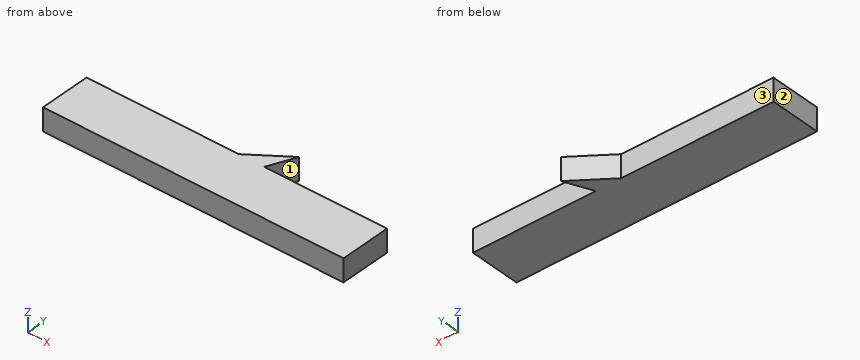
from build123d import *

# Parameters (mm, degrees)
F1_DEPTH = 25


with BuildPart() as f1:
    # F0 (on Top) → F1 (new body)
    with BuildSketch(Plane.XY):
        Polygon((-143.368647, 7.681685), (-52.16566, 7.681685), (25.298358, 63.81616), (-143.368647, 63.81616), align=None)
        Polygon((25.298358, 63.81616), (-52.16566, 7.681685), (189.367071, 7.681685), (189.367071, 63.81616), (53.402534, 63.81616), align=None)
        Polygon((66.434935, 93.625873), (25.298358, 63.81616), (53.402534, 63.81616), align=None)
    extrude(amount=F1_DEPTH)


solid = f1.part
Geometry check sheet. Reference: the model listing, model coordinates, mm. Face numbers are marked on the shaded views. Round coordinates to 2 decimals unless told otherwise and drop trailing zeros. Write each loop counter-clockwise with the first axis right and the second up, starting at its lowest first coordinate (ties: lowest second). Pieces come first, ordered by that corner, then holes. Notation, with made-up numbers: (44.25, 34.5) - (63.25, 34.5) arc R13 cw to (63.25, 55.5) - close; hole circle Ø8 at (56, 83.25). An arc over 180 degrees is marked (long way). One line per item, written item: value.
1. Cross-section at D-D on y = 68. Record the boundary of the cut face in (x, z), and give its area (3 significant figures).
The answers:
outline: (31.07, 0) - (55.23, 0) - (55.23, 25) - (31.07, 25) - close
area: 604 mm^2
2. Scan lines: L1, parallel to Y at x = -62.5, z = 11.25; L2, parallel to X at y = 77, z = 9.25; L3, parallel to X at y = 84, z = 23. Record each from-to range of solid material in increasing order.
The answers:
L1: y = 7.68 to 63.82
L2: x = 43.49 to 59.17
L3: x = 53.15 to 62.23
3. Cross-section at A-A on z = 9.5. Record the boundary of the cut face in (x, y), and give its area (3 significant figures).
The answers:
outline: (-143.37, 7.68) - (189.37, 7.68) - (189.37, 63.82) - (53.4, 63.82) - (66.43, 93.63) - (25.3, 63.82) - (-143.37, 63.82) - close
area: 19,100 mm^2
4. Cross-section at B-B on x = 62.5. Record the boundary of the cut face in (y, z).
The answers:
outline: (7.68, 0) - (63.82, 0) - (63.82, 25) - (7.68, 25) - close; (84.63, 0) - (90.77, 0) - (90.77, 25) - (84.63, 25) - close
5. Cross-section at C-C on x = -54. Record the boundary of the cut face in (y, z).
The answers:
outline: (7.68, 0) - (63.82, 0) - (63.82, 25) - (7.68, 25) - close
6. Depth check by flat-ended pin: pin 1 Ø5 at (x, z) = (60, 19.5) entering from +Y; pin 2 Ø12.5 at (x, z) = (154, 9) entering from +Y. Enter the tip coordinate at first touch or a pass-through.
The answers:
pin 1: stops at y = 90.77
pin 2: stops at y = 63.82
7. Mould release check, pull along Y, two halves, no side actions. Record for the marked faces 1, 2 and 3: released by +Y, released by -Y, zero draft, split by the parting line, or undercut.
The answers:
face 1: undercut
face 2: zero draft
face 3: released by +Y
